For this review, take the finished solid that the model builds, in its own axes (mm). Face numbers are marked on the shaded views. A direction names the side the tool comes from. Coordinates: 2 decimals unless noted, no trailing zeros. Loops run counter-clockwise (first coordinate to the right, second up) from the corner with the lowest first, then second, coordinate; pieces in that order, holes last.
1. Clearance check with flat-ended pins moving along their axes: P1, Ø2, axis at x = 0.5, z = -3, coming from the +Y side; P2, Ø2, axis at y = 0, z = -2.5, coming from the +X side; P3, Ø0.7, axis at y = 0, z = -15, coming from the +X side. State where each tip first meets the part, or that it passes through.
2. Take a section at B-B, the plane z = -6.25. State the section outline as (x, y) points.
3. Mouldability with a two-part tool opening along X and no side actions: class the marked faces 3, 4 and 5 as pulls with the +X half, pulls with the -X half, needs draft (parallel to the pull), parting line crosses it, or undercut.
4. Take a section at A-A, the plane y = 0. State the section outline as (x, z) points.
5. Machinability: for the marked faces 1 and 2, which of the approach directions +Z, -Z, +X, -X, +Y, -Y give a long, thin tool a straight path to every point of the face, cutting with its end or side? Answer none if there is none.
6. To check wall thickness, follow probe 1 along X at (y, z) = (0, -5.5); probe 2 along Y at (x, z) = (1, -15); probe 3 along Y at (x, z) = (1, -5.25). State the ranges of each line that lie inside material, in increasing order.
Autodesk Inventor part; units mm, degrees
ref_plane "YZ Plane" through (0, 0, 0) normal (1, 0, 0) x (0, 1, 0)
ref_plane "XZ Plane" through (0, 0, 0) normal (0, 1, 0) x (-1, 0, 0)
ref_plane "XY Plane" through (0, 0, 0) normal (0, 0, 1) x (1, 0, 0)
sketch "Sketch1" plane through (0, 0, 0) normal (1, 0, 0) x (0, 1, 0)
  line L0 (0, 0) -> (0, -16)
  line L1 (0, -16) -> (4, -16)
  line L2 (2, 0) -> (0, 0)
  line L3 (2, 0) -> (2, -13.7)
  line L4 (2, -13.7) -> (4, -15.7)
  line L5 (4, -15.7) -> (4, -16)
  dimension "d0" = 16
  dimension "d4" = 2
  dimension "d5" = 2.3
  dimension "d6" = 45
  dimension "d7" = 4
revolve "Revolution1" add sketch "Sketch1" angle 360 about axis through (0, 0, 0) along (0, 0, -1)
sketch "Sketch2" plane through (0, 0, -16) normal (0, 0, -1) x (-1, 0, 0)
  line L0 (0, 1.4434) -> (1.25, 0.7217)
  line L1 (1.25, 0.7217) -> (1.25, -0.7217)
  line L2 (1.25, -0.7217) -> (0, -1.4434)
  line L3 (0, -1.4434) -> (-1.25, -0.7217)
  line L4 (-1.25, -0.7217) -> (-1.25, 0.7217)
  line L5 (-1.25, 0.7217) -> (0, 1.4434)
  point P0 (0, 0)
  point P1 (0, 0)
  dimension "d9" = 2.5
extrude "Extrusion1" cut sketch "Sketch2" against normal blind 1.75
thread "Thread1"
chamfer "Chamfer1" distance 0.2 angle 45 1 edges at (0, -2, 0)
properties part number "MM-MMount_to_Motor-CS_Bolt-"
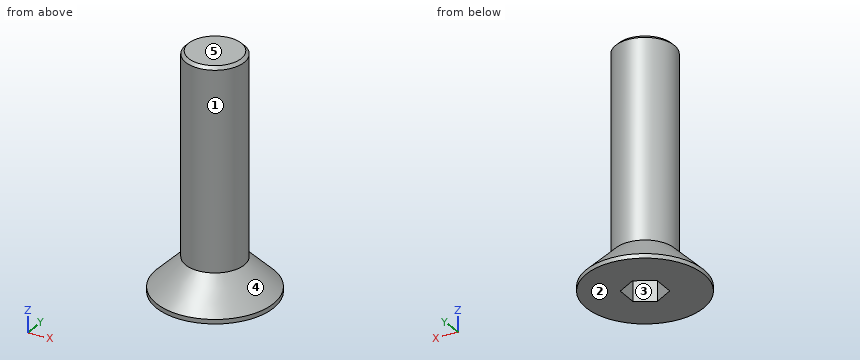
Results list:
1. P1: stops at y = 2
1. P2: stops at x = 2
1. P3: stops at x = 3.65
2. outline: circle Ø4 at (0, 0)
3. face 3: undercut
3. face 4: parting line crosses it
3. face 5: needs draft
4. outline: (-4, -16) - (-1.25, -16) - (-1.25, -14.25) - (1.25, -14.25) - (1.25, -16) - (4, -16) - (4, -15.7) - (2, -13.7) - (2, -0.2) - (1.8, 0) - (-1.8, 0) - (-2, -0.2) - (-2, -13.7) - (-4, -15.7) - close
5. face 1: +Z
5. face 2: -Z, +X, -X, +Y, -Y
6. probe 1: x = -2 to 2
6. probe 2: y = -3.14 to -0.87, 0.87 to 3.14
6. probe 3: y = -1.73 to 1.73
